from build123d import *

# Parameters (mm, degrees)
SKETCH_1_W          = 200
SKETCH_1_H          = 125
EXTRUDE_1_DEPTH     = 2
SKETCH_2_R          = 2
CUT_EXTRUDE_1_DEPTH = 236.858008132
SKETCH_3_R          = 20
SKETCH_3_R_2        = 3
CUT_EXTRUDE_2_DEPTH = 236.858008132
FILLET_1_R          = 20


with BuildPart() as part:
    # Эскиз1 → Бобышка-Вытянуть1 (new body)
    with BuildSketch(Plane(origin=(0, 0, 0), x_dir=(1, 0, 0), z_dir=(0, 1, 0))):
        with Locations((100, 62.5)):
            Rectangle(SKETCH_1_W, SKETCH_1_H)
    extrude(amount=EXTRUDE_1_DEPTH)

    # Эскиз2 → Вырез-Вытянуть1 (cut, through all)
    with BuildSketch(Plane.XZ):
        with Locations(Location((27.25, -6.75, 0), (0, 0, 270))):
            Circle(SKETCH_2_R)
        with Locations(Location((67.25, -6.75, 0), (0, 0, 270))):
            Circle(SKETCH_2_R)
        with Locations(Location((132.75, -6.75, 0), (0, 0, 270))):
            Circle(SKETCH_2_R)
        with Locations(Location((172.75, -6.75, 0), (0, 0, 270))):
            Circle(SKETCH_2_R)
        with Locations(Location((172.75, -52.75, 0), (0, 0, 270))):
            Circle(SKETCH_2_R)
        with Locations(Location((132.75, -52.75, 0), (0, 0, 270))):
            Circle(SKETCH_2_R)
        with Locations(Location((132.75, -72.25, 0), (0, 0, 270))):
            Circle(SKETCH_2_R)
        with Locations(Location((172.75, -72.25, 0), (0, 0, 270))):
            Circle(SKETCH_2_R)
        with Locations(Location((132.75, -118.25, 0), (0, 0, 270))):
            Circle(SKETCH_2_R)
        with Locations(Location((172.75, -118.25, 0), (0, 0, 270))):
            Circle(SKETCH_2_R)
        with Locations(Location((27.25, -52.75, 0), (0, 0, 270))):
            Circle(SKETCH_2_R)
        with Locations(Location((67.25, -52.75, 0), (0, 0, 270))):
            Circle(SKETCH_2_R)
        with Locations(Location((27.25, -72.25, 0), (0, 0, 270))):
            Circle(SKETCH_2_R)
        with Locations(Location((67.25, -72.25, 0), (0, 0, 270))):
            Circle(SKETCH_2_R)
        with Locations(Location((67.25, -118.25, 0), (0, 0, 270))):
            Circle(SKETCH_2_R)
        with Locations(Location((27.25, -118.25, 0), (0, 0, 270))):
            Circle(SKETCH_2_R)
    extrude(amount=-CUT_EXTRUDE_1_DEPTH, mode=Mode.SUBTRACT)

    # Эскиз3 → Вырез-Вытянуть2 (cut, through all)
    with BuildSketch(Plane.XZ):
        with Locations(Location((47.25, -29.75, 0), (0, 0, 270))):
            Circle(SKETCH_3_R)
        with Locations(Location((152.75, -29.75, 0), (0, 0, 270))):
            Circle(SKETCH_3_R)
        with Locations(Location((152.75, -95.25, 0), (0, 0, 270))):
            Circle(SKETCH_3_R)
        with Locations(Location((47.25, -95.25, 0), (0, 0, 270))):
            Circle(SKETCH_3_R)
        with Locations(Location((100, -62.5, 0), (0, 0, 270))):
            Circle(SKETCH_3_R_2)
        with Locations(Location((100, -29.75, 0), (0, 0, 270))):
            Circle(SKETCH_3_R_2)
        with Locations(Location((100, -95.25, 0), (0, 0, 270))):
            Circle(SKETCH_3_R_2)
        with Locations(Location((100, -13.375, 0), (0, 0, 270))):
            Circle(SKETCH_3_R_2)
        with Locations(Location((100, -46.125, 0), (0, 0, 270))):
            Circle(SKETCH_3_R_2)
        with Locations(Location((100, -78.875, 0), (0, 0, 270))):
            Circle(SKETCH_3_R_2)
        with Locations(Location((100, -111.625, 0), (0, 0, 270))):
            Circle(SKETCH_3_R_2)
    extrude(amount=-CUT_EXTRUDE_2_DEPTH, mode=Mode.SUBTRACT)

    # Скругление1
    fillet_1_edges = [part.edges().sort_by_distance(p)[0] for p in [
        (0, 1, -125),
        (200, 1, -125),
        (200, 1, 0),
        (0, 1, 0),
    ]]
    fillet(fillet_1_edges, radius=FILLET_1_R)


solid = part.part
Read the model definition and answer for the solid it produces. Units are mm, in the model's axes. Round coordinates to 2 decimals unless told otherwise and drop trailing zeros. Order: outer loops, then holes, each group sorted by start corner. A loop starts at its lowest first (then second) coordinate and runs counter-clockwise, first axis right, second up.
1) The part is cut by section D-D on z = -6.75. Write down the section's boundary in (x, y), plus the area to 3 significant figures.
2) The mould has two halves that part along Z. Classify faces 1 (the face through (193.986, 1.014, -119.297)), 2 (the face through (25.476, 0.986, -73.173)), 3 (the face through (48.13, 0.99, -75.27)): released by +Z, released by -Z, zero draft, split by the parting line, or undercut.
3) The part is cut by section C-C on y = 1.15. Give the number of separate pieces and of enclosed holes in the cut face, plus the area to 3 significant figures.
4) A flat-ended cylindrical pin translates along its axis: pin 1 (3.5 mm diameter, centred on x = 27.25, z = -52.75, fed in from +Y). Find the tip coordinate at first contact, or state that the pin passes through.
5) The part is cut by section B-B on z = -95.25. Write down the section's boundary in (x, y).
6) The part is cut by section A-A on x = 47.25. Write down the section's boundary in (y, z), plus the area to 3 significant figures.
7) Straight lines are drawn through the part: L1, parallel to X at y = 0.7, z = -29.75; L2, parallel to X at y = 1.5, z = -72.25; L3, parallel to Z at x = 151.5, y = 1.9. For each, find the intervals that lie inside material, in ascending order.
Resolved:
1. outline: (5.02, 0) - (25.25, 0) - (25.25, 2) - (5.02, 2) - close; (29.25, 0) - (65.25, 0) - (65.25, 2) - (29.25, 2) - close; (69.25, 0) - (130.75, 0) - (130.75, 2) - (69.25, 2) - close; (134.75, 0) - (170.75, 0) - (170.75, 2) - (134.75, 2) - close; (174.75, 0) - (194.98, 0) - (194.98, 2) - (174.75, 2) - close
1. area: 348 mm2
2. face 1: released by -Z
2. face 2: undercut
2. face 3: undercut
3. separate pieces: 1
3. enclosed holes: 27
3. area: 19,200 mm2
4. pin 1: passes through
5. outline: (0, 0) - (27.25, 0) - (27.25, 2) - (0, 2) - close; (67.25, 0) - (97, 0) - (97, 2) - (67.25, 2) - close; (103, 0) - (132.75, 0) - (132.75, 2) - (103, 2) - close; (172.75, 0) - (200, 0) - (200, 2) - (172.75, 2) - close
6. outline: (0, -125) - (2, -125) - (2, -115.25) - (0, -115.25) - close; (0, -75.25) - (2, -75.25) - (2, -49.75) - (0, -49.75) - close; (0, -9.75) - (2, -9.75) - (2, 0) - (0, 0) - close
6. area: 90.0 mm2
7. L1: x = 0 to 27.25, 67.25 to 97, 103 to 132.75, 172.75 to 200
7. L2: x = 0 to 25.25, 29.25 to 65.25, 69.25 to 130.75, 134.75 to 170.75, 174.75 to 200
7. L3: z = -125 to -115.21, -75.29 to -49.71, -9.79 to 0
